```python
from build123d import *

# Parameters (mm, degrees)
BOSS_EXTRUDE1_DEPTH  = 21
SKETCH4_W            = 42
SKETCH4_H            = 5
BOSS_EXTRUDE2_DEPTH  = 21
SKETCH5_W            = 21
SKETCH5_H            = 5
BOSS_EXTRUDE3_DEPTH  = 5
SKETCH7_W            = 5.022630365
SKETCH7_H            = 30.4
BOSS_EXTRUDE4_DEPTH  = 21
SKETCH8_W            = 26
SKETCH8_H            = 35.4
BOSS_EXTRUDE5_DEPTH  = 5
SKETCH9_W            = 26
SKETCH9_H            = 5
BOSS_EXTRUDE6_DEPTH  = 16
SKETCH10_W           = 16
SKETCH10_H           = 30.4
BOSS_EXTRUDE7_DEPTH  = 5
SKETCH11_W           = 21
SKETCH11_H           = 5
BOSS_EXTRUDE9_DEPTH  = 30.4
SKETCH13_W           = 21
SKETCH13_H           = 4.993745126
BOSS_EXTRUDE10_DEPTH = 30.4
SKETCH15_W           = 30.4
SKETCH15_H           = 5
BOSS_EXTRUDE11_DEPTH = 21
SKETCH18_W           = 5
SKETCH18_H           = 30.4
BOSS_EXTRUDE12_DEPTH = 21
SKETCH19_W           = 4.993745126
SKETCH19_H           = 30.4
BOSS_EXTRUDE13_DEPTH = 21
SKETCH21_W           = 21
SKETCH21_H           = 21
SKETCH21_W_2         = 20
SKETCH21_H_2         = 20
BOSS_EXTRUDE19_DEPTH = 30.4
SKETCH22_R           = 2.5
CUT_EXTRUDE1_DEPTH   = 47.02263
SKETCH24_R           = 2.5
CUT_EXTRUDE2_DEPTH   = 5.5
SKETCH25_R           = 2.5
CUT_EXTRUDE3_DEPTH   = 5
SKETCH26_R           = 2.5
CUT_EXTRUDE4_DEPTH   = 57.4
SKETCH28_W           = 21
SKETCH28_H           = 30.4
CUT_EXTRUDE5_DEPTH   = 0.006255


with BuildPart() as part:
    # Sketch2 → Boss-Extrude1 (new body)
    with BuildSketch(Plane(origin=(0, 0, 0), x_dir=(0, 0, -1), z_dir=(1, 0, 0))):
        Polygon((-17.7, 17.7), (17.7, 17.7), (17.7, -17.7), (12.7, -17.7), (12.7, -12.7), (12.7, 12.7), (-12.7, 12.7), (-12.7, -12.7), (-12.7, -17.7), (-17.7, -17.7), align=None)
    extrude(amount=BOSS_EXTRUDE1_DEPTH)

    # Sketch4 → Boss-Extrude2 (add)
    with BuildSketch(Plane.XY.offset(17.7)):
        with Locations((0, -15.2)):
            Rectangle(SKETCH4_W, SKETCH4_H)
    extrude(amount=BOSS_EXTRUDE2_DEPTH)

    # Sketch5 → Boss-Extrude3 (add)
    with BuildSketch(Plane(origin=(0, 0, 17.7), x_dir=(-1, 0, 0), z_dir=(0, 0, -1))):
        with Locations((10.5, -15.2)):
            Rectangle(SKETCH5_W, SKETCH5_H)
    extrude(amount=BOSS_EXTRUDE3_DEPTH)

    # Sketch7 → Boss-Extrude4 (add)
    with BuildSketch(Plane.XY.offset(17.7)):
        with Locations((2.511315183, 2.5)):
            Rectangle(SKETCH7_W, SKETCH7_H)
    extrude(amount=BOSS_EXTRUDE4_DEPTH)

    # Sketch8 → Boss-Extrude5 (add)
    with BuildSketch(Plane.ZY.offset(21)):
        with Locations((25.7, 0)):
            Rectangle(SKETCH8_W, SKETCH8_H)
    extrude(amount=BOSS_EXTRUDE5_DEPTH)

    # Sketch9 → Boss-Extrude6 (add)
    with BuildSketch(Plane.ZY.offset(26)):
        with Locations((25.7, -15.2)):
            Rectangle(SKETCH9_W, SKETCH9_H)
    extrude(amount=BOSS_EXTRUDE6_DEPTH)

    # Sketch10 → Boss-Extrude7 (add)
    with BuildSketch(Plane(origin=(0, 0, 12.7), x_dir=(-1, 0, 0), z_dir=(0, 0, -1))):
        with Locations((34, 2.5)):
            Rectangle(SKETCH10_W, SKETCH10_H)
    extrude(amount=-BOSS_EXTRUDE7_DEPTH)

    # Sketch11 → Boss-Extrude9 (add)
    with BuildSketch(Plane(origin=(0, 0, 12.7), x_dir=(-1, 0, 0), z_dir=(0, 0, -1))):
        with Locations((31.5, 15.2)):
            Rectangle(SKETCH11_W, SKETCH11_H)
    extrude(amount=BOSS_EXTRUDE9_DEPTH)

    # Sketch13 → Boss-Extrude10 (add)
    with BuildSketch(Plane.XZ.offset(-12.7)):
        with Locations((-31.5, -15.203127437)):
            Rectangle(SKETCH13_W, SKETCH13_H)
    extrude(amount=BOSS_EXTRUDE10_DEPTH)

    # Sketch15 → Boss-Extrude11 (add)
    with BuildSketch(Plane(origin=(-21, 0, 0), x_dir=(0, 0, -1), z_dir=(1, 0, 0))):
        with Locations((2.5, 15.2)):
            Rectangle(SKETCH15_W, SKETCH15_H)
    extrude(amount=BOSS_EXTRUDE11_DEPTH)

    # Sketch18 → Boss-Extrude12 (add)
    with BuildSketch(Plane(origin=(-21, 0, 0), x_dir=(0, 0, -1), z_dir=(1, 0, 0))):
        with Locations((-36.2, 2.5)):
            Rectangle(SKETCH18_W, SKETCH18_H)
    extrude(amount=BOSS_EXTRUDE12_DEPTH)

    # Sketch19 → Boss-Extrude13 (add)
    with BuildSketch(Plane(origin=(-21, 0, 0), x_dir=(0, 0, -1), z_dir=(1, 0, 0))):
        with Locations((15.203127437, -2.5)):
            Rectangle(SKETCH19_W, SKETCH19_H)
    extrude(amount=BOSS_EXTRUDE13_DEPTH)

    # Sketch21 → Boss-Extrude19 (add)
    with BuildSketch(Plane(origin=(0, 17.7, 0), x_dir=(1, 0, 0), z_dir=(0, 1, 0))):
        with Locations((-10.5, -23.2)):
            Rectangle(SKETCH21_W, SKETCH21_H)
        with Locations((-10.5, -23.2)):
            Rectangle(SKETCH21_W_2, SKETCH21_H_2, mode=Mode.SUBTRACT)
    extrude(amount=-BOSS_EXTRUDE19_DEPTH)

    # Sketch22 → Cut-Extrude1 (cut)
    with BuildSketch(Plane(origin=(5.022630365, 0, 0), x_dir=(0, 0, -1), z_dir=(1, 0, 0))):
        with Locations((-23.2, 10.1)):
            Circle(SKETCH22_R)
        with Locations((-23.2, -5.1)):
            Circle(SKETCH22_R)
    extrude(amount=-CUT_EXTRUDE1_DEPTH, mode=Mode.SUBTRACT)

    # Sketch24 → Cut-Extrude2 (cut)
    with BuildSketch(Plane.XY.offset(38.7)):
        with Locations((-10.488684817, 10.1)):
            Circle(SKETCH24_R)
        with Locations((-10.488684817, -5.1)):
            Circle(SKETCH24_R)
    extrude(amount=-CUT_EXTRUDE2_DEPTH, mode=Mode.SUBTRACT)

    # Sketch25 → Cut-Extrude3 (cut)
    with BuildSketch(Plane(origin=(0, 17.7, 0), x_dir=(1, 0, 0), z_dir=(0, 1, 0))):
        with Locations((-10.5, 2.25)):
            Circle(SKETCH25_R)
        with Locations((9.5, 2.25)):
            Circle(SKETCH25_R)
        with Locations((-30.5, 2.25)):
            Circle(SKETCH25_R)
    extrude(amount=-CUT_EXTRUDE3_DEPTH, mode=Mode.SUBTRACT)

    # Sketch26 → Cut-Extrude4 (cut, through all)
    with BuildSketch(Plane(origin=(0, 0, -17.7), x_dir=(-1, 0, 0), z_dir=(0, 0, -1))):
        with Locations((-13.5, 0)):
            Circle(SKETCH26_R)
        with Locations((34.5, 0)):
            Circle(SKETCH26_R)
    extrude(amount=-CUT_EXTRUDE4_DEPTH, mode=Mode.SUBTRACT)

    # Sketch28 → Cut-Extrude5 (cut)
    with BuildSketch(Plane.XY.offset(-12.7)):
        with Locations((10.5, -2.5)):
            Rectangle(SKETCH28_W, SKETCH28_H)
    extrude(amount=-CUT_EXTRUDE5_DEPTH, mode=Mode.SUBTRACT)


solid = part.part
```
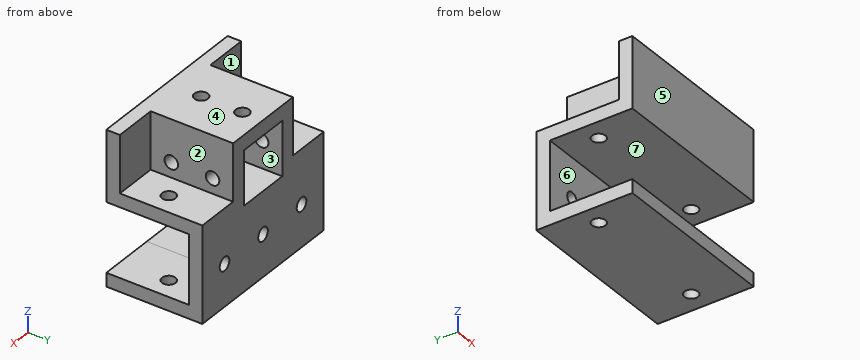
The model under review builds one solid part; all positions refer to its coordinate system, in mm. Face numbers are marked on the shaded views. A direction names the side the tool comes from. Round coordinates to 2 decimals unless told otherwise and drop trailing zeros. Loops run counter-clockwise (first coordinate to the right, second up) from the corner with the lowest first, then second, coordinate; pieces in that order, holes last. Notation, with made-up numbers: M -10,-23 L 43,-23 A20 cw 43,9 Z; hole C -4.5,4.5 d10. An arc over 180 degrees is marked long. Put each result on its own line as item: value.
Q1. Consider section D-D, the plane z = 23.2. Give the boundary of the cut face in (x, y), then the cut area to 3 significant figures.
Result set:
outline: M -42,-17.7 L 21,-17.7 L 21,-12.7 L 5.02,-12.7 L 5.02,-7.6 L -0.5,-7.6 L -0.5,-12.7 L -20.5,-12.7 L -20.5,-7.6 L -26,-7.6 L -26,-12.7 L -42,-12.7 Z; M -26,-2.6 L -20.5,-2.6 L -20.5,7.6 L -26,7.6 Z; M -26,12.6 L -20.5,12.6 L -20.5,17.7 L -26,17.7 Z; M -0.5,-2.6 L 5.02,-2.6 L 5.02,7.6 L -0.5,7.6 Z; M -0.5,12.6 L 5.02,12.6 L 5.02,17.7 L -0.5,17.7 Z
area: 540 mm²
Q2. To check wall thickness, follow L1, parallel to Y at x = -24.45, z = 23.2; L2, parallel to Z at x = -2.5, y = 8; L3, parallel to Z at x = 8.5, y = 5. State the ranges of each line that lie inside material, in increasing order.
Result set:
L1: y = -17.7 to -7.6, -2.6 to 7.6, 12.6 to 17.7
L2: z = -17.7 to -12.71, 12.7 to 13.2, 33.2 to 38.7
L3: z = -17.7 to -12.71, 12.7 to 17.7
Q3. Consider section A-A, the plane y = 0. Count the separate pieces of the cut face and the enclosed holes in it, then the cut area to 3 significant figures.
Result set:
separate pieces: 6
enclosed holes: 1
area: 781 mm²
Q4. Consider section C-C, the plane y = 4.5. Give the boundary of the cut face in (x, z), then the cut area to 3 significant figures.
Result set:
outline: M -42,-17.7 L 21,-17.7 L 21,-12.71 L -42,-12.71 Z; M -42,12.7 L 21,12.7 L 21,17.7 L 5.02,17.7 L 5.02,38.7 L -26,38.7 L -26,17.7 L -42,17.7 Z; hole M -20.5,13.2 L -0.5,13.2 L -0.5,33.2 L -20.5,33.2 Z
area: 881 mm²
Q5. For pin 1 (8 mm diameter, centred on y = 10.1, z = 23.2, fed in from +X); pin 2 (12 mm diameter, centred on y = -1.5, z = 29, fed in from -X); pin 3 (7.5 mm diameter, centred on x = -14.5, z = -1.5, fed in from -Y); pin 4 (3 mm diameter, centred on x = 13.5, y = 0, fed in from -Z) (1 decimal), all flat-tipped, find the tip position at first contact; note any pin that passes through.
Result set:
pin 1: stops at x = 5.02
pin 2: stops at x = -26
pin 3: stops at y = 12.7
pin 4: passes through
Q6. Mouldability with a two-part tool opening along Z and no side actions: class the marked faces 4, 5, 6 and 7 as released by +Z, released by -Z, zero draft, split by the parting line, or undercut.
Result set:
face 4: released by +Z
face 5: zero draft
face 6: undercut
face 7: undercut
Q7. Machinability: for the marked faces 1, 2 and 3, which of the approach directions +Z, -Z, +X, -X, +Y, -Y give a long, thin tool a straight path to every point of the face, cutting with its end or side? Answer none if there is none.
Result set:
face 1: +Z, -X, +Y
face 2: +Z, +X, +Y
face 3: +Y
Q8. Consider section B-B, the plane x = -36. Give the boundary of the cut face in (y, z), then the cut area to 3 significant figures.
Result set:
outline: M -17.7,-17.7 L -2,-17.7 L -2,-12.71 L -17.7,-12.71 Z; M -17.7,12.7 L -2,12.7 L -2,17.7 L -12.7,17.7 L -12.7,38.7 L -17.7,38.7 Z; M 2,-17.7 L 17.7,-17.7 L 17.7,17.7 L 2,17.7 L 2,12.7 L 12.7,12.7 L 12.7,-12.71 L 2,-12.71 Z
area: 546 mm²
